Geometry check sheet. Reference: the model listing, model coordinates, mm. Face numbers are marked on the shaded views. A direction names the side the tool comes from. Round coordinates to 2 decimals unless told otherwise and drop trailing zeros. Order: outer loops, then holes, each group sorted by start corner. A loop starts at its lowest first (then second) coordinate and runs counter-clockwise, first axis right, second up.
(1) Cross-section at D-D on y = 30. Enter the section's corners in (x, z), and give its area (3 significant figures).
(2) Gauge pin test, flat ends, axial feed: P1, Ø9.5, axis at x = -15.4, z = -15.4, coming from the -Y side; P2, Ø2.5, axis at x = 15.6, z = -15.4, coming from the -Y side; P3, Ø6.5, axis at x = 16.5, z = -15, coming from the +Y side; P4, Ø3.5, axis at x = 15.6, z = -15.4, coming from the +Y side. Record the tip position at first contact, or that the pin passes through.
(3) Draft check along Z on the marked faces 3, 4 and 5. Enter one of: pulls with the +Z half, pulls with the -Z half, needs draft (parallel to the pull), parting line crosses it, or undercut.
(4) Cross-section at C-C on z = 15.6. Enter the section's corners in (x, y).
(5) Cross-section at A-A on y = 8. Enter the section's corners in (x, z), and give its area (3 significant figures).
(6) Thickness scan on L1, parallel to X at y = 49.75, z = 15.6; L2, parallel to Y at x = 23.3, z = 0; L3, parallel to X at y = 52.25, z = 0. Record the ranges inside material, lowest first.
(7) Cross-section at B-B on x = 0. Enter the section's corners in (y, z).
(8) Set-up check for the marked faces 1 and 2: record each of +Z, -Z, +X, -X, +Y, -Y from which the full face is reachable in a straight line by a thin tool's end or side.
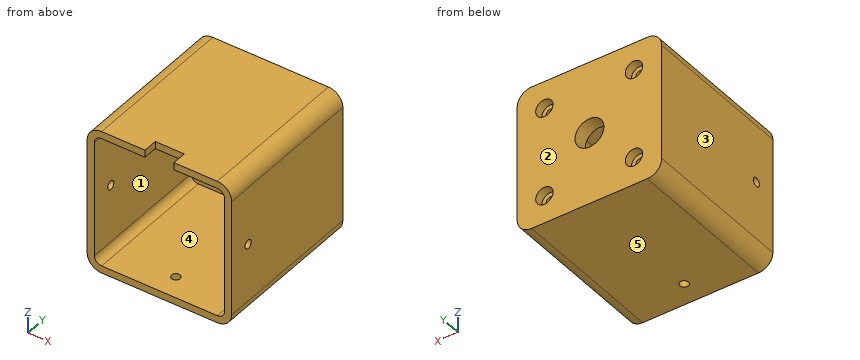
from build123d import *

# Parameters (mm, degrees)
SKETCH1_W           = 50
SKETCH1_H           = 50
SKETCH1_W_2         = 45
SKETCH1_H_2         = 45
BOSS_EXTRUDE1_DEPTH = 47
SKETCH3_W           = 50
SKETCH3_H           = 50
BOSS_EXTRUDE3_DEPTH = 7
SKETCH5_R           = 11.5
CUT_EXTRUDE1_DEPTH  = 2
SKETCH6_R           = 5
CUT_EXTRUDE2_DEPTH  = 61.42350536
FILLET2_R           = 5
FILLET3_R           = 5
FILLET4_R           = 5
FILLET5_R           = 5
FILLET7_R           = 2.5
FILLET8_R           = 2.5
FILLET9_R           = 2.5
FILLET10_R          = 2.5
SKETCH9_W           = 10
SKETCH9_H           = 5
CUT_EXTRUDE5_DEPTH  = 13
SKETCH10_R          = 1.5
CUT_EXTRUDE6_DEPTH  = 10
CIRPATTERN1_COUNT   = 4
HOLE1_D             = 3
HOLE1_DEPTH         = 12
HOLE1_CBORE_D       = 6
HOLE1_CBORE_DEPTH   = 3


with BuildPart() as part:
    # Sketch1 → Boss-Extrude1 (new body)
    with BuildSketch(Plane(origin=(0, 0, 0), x_dir=(1, 0, 0), z_dir=(0, 1, 0))):
        Rectangle(SKETCH1_W, SKETCH1_H)
        Rectangle(SKETCH1_W_2, SKETCH1_H_2, mode=Mode.SUBTRACT)
    extrude(amount=BOSS_EXTRUDE1_DEPTH)

    # Sketch3 → Boss-Extrude3 (add)
    with BuildSketch(Plane(origin=(0, 47, 0), x_dir=(1, 0, 0), z_dir=(0, 1, 0))):
        Rectangle(SKETCH3_W, SKETCH3_H)
    extrude(amount=BOSS_EXTRUDE3_DEPTH)

    # Sketch5 → Cut-Extrude1 (cut)
    with BuildSketch(Plane.XZ.offset(-47)):
        with Locations(Location((0, 0, 0), (0, 0, 270))):
            Circle(SKETCH5_R)
    extrude(amount=-CUT_EXTRUDE1_DEPTH, mode=Mode.SUBTRACT)

    # Sketch6 → Cut-Extrude2 (cut, through all)
    with BuildSketch(Plane.XZ.offset(-49)):
        with Locations(Location((0, 0, 0), (0, 0, 270))):
            Circle(SKETCH6_R)
    extrude(amount=-CUT_EXTRUDE2_DEPTH, mode=Mode.SUBTRACT)

    # Fillet2
    fillet2_edges = [part.edges().sort_by_distance(p)[0] for p in [
        (25, 27, 25),
    ]]
    fillet(fillet2_edges, radius=FILLET2_R)

    # Fillet3
    fillet3_edges = [part.edges().sort_by_distance(p)[0] for p in [
        (25, 27, -25),
    ]]
    fillet(fillet3_edges, radius=FILLET3_R)

    # Fillet4
    fillet4_edges = [part.edges().sort_by_distance(p)[0] for p in [
        (-25, 27, -25),
    ]]
    fillet(fillet4_edges, radius=FILLET4_R)

    # Fillet5
    fillet5_edges = [part.edges().sort_by_distance(p)[0] for p in [
        (-25, 27, 25),
    ]]
    fillet(fillet5_edges, radius=FILLET5_R)

    # Fillet7
    fillet7_edges = [part.edges().sort_by_distance(p)[0] for p in [
        (-22.5, 23.5, 22.5),
    ]]
    fillet(fillet7_edges, radius=FILLET7_R)

    # Fillet8
    fillet8_edges = [part.edges().sort_by_distance(p)[0] for p in [
        (22.5, 23.5, 22.5),
    ]]
    fillet(fillet8_edges, radius=FILLET8_R)

    # Fillet9
    fillet9_edges = [part.edges().sort_by_distance(p)[0] for p in [
        (22.5, 23.5, -22.5),
    ]]
    fillet(fillet9_edges, radius=FILLET9_R)

    # Fillet10
    fillet10_edges = [part.edges().sort_by_distance(p)[0] for p in [
        (-22.5, 23.5, -22.5),
    ]]
    fillet(fillet10_edges, radius=FILLET10_R)

    # Sketch9 → Cut-Extrude5 (cut)
    with BuildSketch(Plane.XY.offset(25)):
        with Locations((0, 2.5)):
            Rectangle(SKETCH9_W, SKETCH9_H)
    extrude(amount=-CUT_EXTRUDE5_DEPTH, mode=Mode.SUBTRACT)

    # Sketch10 → Cut-Extrude6 (cut)
    with BuildSketch(Plane(origin=(25, 0, 0), x_dir=(0, 0, -1), z_dir=(1, 0, 0))):
        with Locations((0, 8)):
            Circle(SKETCH10_R)
    cut_extrude6 = extrude(amount=-CUT_EXTRUDE6_DEPTH, mode=Mode.SUBTRACT)

    # CirPattern1: Cut-Extrude6 ×4 about axis, 1 skipped
    cirpattern1_axis = Axis((0, 54, 0), (0, -1, 0))
    add([cut_extrude6.rotate(cirpattern1_axis, i * 360 / CIRPATTERN1_COUNT) for i in range(1, CIRPATTERN1_COUNT) if i not in (1,)], mode=Mode.SUBTRACT)

    # Hole1
    with Locations(Plane(origin=(-15.4, 54, -15.4), x_dir=(0, 0, 1), z_dir=(0, 1, 0))):
        with Locations((0, 0), (0, 31), (31, 31), (31, 0)):
            CounterBoreHole(HOLE1_D / 2, HOLE1_CBORE_D / 2, HOLE1_CBORE_DEPTH, depth=HOLE1_DEPTH)


solid = part.part
Found:
1. outline: (-25, -20) arc R5 ccw to (-20, -25) - (20, -25) arc R5 ccw to (25, -20) - (25, 20) arc R5 ccw to (20, 25) - (-20, 25) arc R5 ccw to (-25, 20) - close; hole (-22.5, -20) arc R2.5 ccw to (-20, -22.5) - (20, -22.5) arc R2.5 ccw to (22.5, -20) - (22.5, 20) arc R2.5 ccw to (20, 22.5) - (-20, 22.5) arc R2.5 ccw to (-22.5, 20) - close
1. area: 459 mm2
2. P1: stops at y = 47
2. P2: passes through
2. P3: stops at y = 54
2. P4: stops at y = 51
3. face 3: needs draft
3. face 4: undercut
3. face 5: pulls with the -Z half
4. outline: (-25, 0) - (-22.5, 0) - (-22.5, 47) - (-16.9, 47) - (-16.9, 51) - (-18.4, 51) - (-18.4, 54) - (-25, 54) - close; (-13.9, 47) - (14.1, 47) - (14.1, 51) - (12.6, 51) - (12.6, 54) - (-12.4, 54) - (-12.4, 51) - (-13.9, 51) - close; (17.1, 47) - (22.5, 47) - (22.5, 0) - (25, 0) - (25, 54) - (18.6, 54) - (18.6, 51) - (17.1, 51) - close
5. outline: (-25, -20) arc R5 ccw to (-20, -25) - (-1.5, -25) - (-1.5, -22.5) - (-20, -22.5) arc R2.5 cw to (-22.5, -20) - (-22.5, -1.5) - (-25, -1.5) - close; (-25, 1.5) - (-22.5, 1.5) - (-22.5, 20) arc R2.5 cw to (-20, 22.5) - (20, 22.5) arc R2.5 cw to (22.5, 20) - (22.5, 1.5) - (25, 1.5) - (25, 20) arc R5 ccw to (20, 25) - (-20, 25) arc R5 ccw to (-25, 20) - close; (1.5, -25) - (20, -25) arc R5 ccw to (25, -20) - (25, -1.5) - (22.5, -1.5) - (22.5, -20) arc R2.5 cw to (20, -22.5) - (1.5, -22.5) - close
5. area: 436 mm2
6. L1: x = -25 to -16.9, -13.9 to 14.1, 17.1 to 25
6. L2: y = 0 to 6.5, 9.5 to 54
6. L3: x = -25 to -5, 5 to 25
7. outline: (0, -25) - (6.5, -25) - (6.5, -22.5) - (0, -22.5) - close; (5, 22.5) - (47, 22.5) - (47, 11.5) - (49, 11.5) - (49, 5) - (54, 5) - (54, 25) - (5, 25) - close; (9.5, -25) - (54, -25) - (54, -5) - (49, -5) - (49, -11.5) - (47, -11.5) - (47, -22.5) - (9.5, -22.5) - close
8. face 1: -Y
8. face 2: +Z, -Z, +X, -X, +Y
